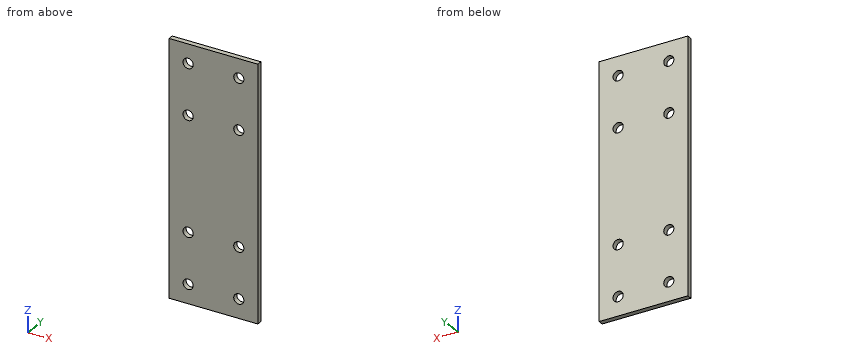
Autodesk Fusion 360 part; units mm, degrees
sketch "Sketch1" plane through (0, 0, 0) normal (0, 1, 0) x (1, 0, 0)
  line L0 (-17.5, 50) -> (17.5, 50)
  line L1 (17.5, 50) -> (17.5, -50)
  line L2 (17.5, -50) -> (-17.5, -50)
  line L3 (-17.5, -50) -> (-17.5, 50)
  circle A0 centre (-10, 42.5) radius 2
  circle A1 centre (10, 42.5) radius 2
  circle A2 centre (-10, 22.5) radius 2
  circle A3 centre (10, 22.5) radius 2
  line L4 (1.75, 0) -> (22.5, 0)
  circle A4 centre (-10, -42.5) radius 2
  circle A5 centre (10, -42.5) radius 2
  circle A6 centre (10, -22.5) radius 2
  circle A7 centre (-10, -22.5) radius 2
  dimension "d1" = 35
  dimension "d2" = 100
  dimension "d3" = 4
  dimension "d6" = 20
  dimension "d7" = -20
  dimension "d8" = 7.5
  dimension "d9" = 7.5
extrude "Extrude1" add sketch "Sketch1" along normal blind 2
equation "d9 = d8"
Can you work these out from the model? Positions are in its coordinate system, mm. Round coordinates to 2 decimals unless told otherwise and drop trailing zeros. Write each loop counter-clockwise with the first axis right and the second up, starting at its lowest first coordinate (ties: lowest second). Pieces come first, ordered by that corner, then holes. Notation, with made-up numbers: (-1, 54) - (20, 54) arc R17 cw to (20, 84) - close; hole circle Ø6 at (54.25, 71.5). An arc over 180 degrees is marked (long way). Write each question's results on one line, items separated by ' | '. Start each with the question number.
1) Suppose I cut it at A-A (y = 0.5). Give the number of separate pieces and of enclosed holes in the cut face, and give its area (3 significant figures).
2) Please list where these lines run through material, in increasing order: line 1 (X direction, y = 1.55, z = 42.5); line 2 (Z direction, x = 10, y = 1.4); line 3 (Z direction, x = 9, y = 0.25).
3) Suppose I cut it at C-C (x = -10). List the corners of the cut face in (y, z) for me, and give its area (3 significant figures).
4) Suppose I cut it at B-B (z = -42.5). List the corners of the cut face in (x, y) for me, and give its area (3 significant figures).
Here are the results:
1) separate pieces: 1 | enclosed holes: 8 | area: 3,400 mm2
2) line 1: x = -17.5 to -12, -8 to 8, 12 to 17.5 | line 2: z = -50 to -44.5, -40.5 to -24.5, -20.5 to 20.5, 24.5 to 40.5, 44.5 to 50 | line 3: z = -50 to -44.23, -40.77 to -24.23, -20.77 to 20.77, 24.23 to 40.77, 44.23 to 50
3) outline: (0, -50) - (2, -50) - (2, -44.5) - (0, -44.5) - close; (0, -40.5) - (2, -40.5) - (2, -24.5) - (0, -24.5) - close; (0, -20.5) - (2, -20.5) - (2, 20.5) - (0, 20.5) - close; (0, 24.5) - (2, 24.5) - (2, 40.5) - (0, 40.5) - close; (0, 44.5) - (2, 44.5) - (2, 50) - (0, 50) - close | area: 168 mm2
4) outline: (-17.5, 0) - (-12, 0) - (-12, 2) - (-17.5, 2) - close; (-8, 0) - (8, 0) - (8, 2) - (-8, 2) - close; (12, 0) - (17.5, 0) - (17.5, 2) - (12, 2) - close | area: 54.0 mm2
